from build123d import *

# Parameters (mm, degrees)
SKETCH1_R          = 20
EXTRUDE1_DEPTH     = 40
SKETCH2_R          = 2.5
SKETCH4_R          = 18
CUT_EXTRUDE1_DEPTH = 38
FILLET1_R          = 0.75
FILLET2_R          = 0.75
SCALE1_SCALE       = 2.5
SCALE2_SCALE       = 1.2


with BuildPart() as part:
    # Sketch1 → Extrude1 (new body)
    with BuildSketch(Plane(origin=(0, 0, 0), x_dir=(1, 0, 0), z_dir=(0, 1, 0))):
        Circle(SKETCH1_R)
    extrude(amount=EXTRUDE1_DEPTH)

    # Sweep1: sweep along a path in Sketch3
    with BuildLine(Plane.XY) as sweep1_path:
        Line((0, 30.773001508), (21.65, 30.773001508))
        ThreePointArc((21.65, 30.773001508), (33.01, 19.413001508), (21.65, 8.053001508))
        Line((21.65, 8.053001508), (0, 8.053001508))
    # Sketch2 → Sweep1 (sweep)
    with BuildSketch(Plane(origin=(0, 0, 0), x_dir=(0, 0, -1), z_dir=(1, 0, 0))):
        with Locations((0, 33.273001508)):
            Circle(SKETCH2_R)
    sweep(path=sweep1_path.line)

    # Sketch4 → Cut-Extrude1 (cut)
    with BuildSketch(Plane(origin=(0, 40, 0), x_dir=(-1, 0, 0), z_dir=(0, 1, 0))):
        Circle(SKETCH4_R)
    extrude(amount=-CUT_EXTRUDE1_DEPTH, mode=Mode.SUBTRACT)

    # Fillet1
    fillet1_edges = [part.edges().sort_by_distance(p)[0] for p in [
        (18, 40, 0),
        (-20, 40, 0),
    ]]
    fillet(fillet1_edges, radius=FILLET1_R)

    # Fillet2
    fillet2_edges = [part.edges().sort_by_distance(p)[0] for p in [
        (18, 2, 0),
    ]]
    fillet(fillet2_edges, radius=FILLET2_R)


with BuildPart() as part_1:
    # Scale1: scaled about (2.200885097, 16.795438051, 2.029e-06)
    add(part.part.scale(SCALE1_SCALE).moved(Location((-3.301327645, -25.193157077, -3.043e-06))))


with BuildPart() as part_2:
    # Scale2: scaled about (2.200885096, 16.795438052, 2.029e-06)
    add(part_1.part.scale(SCALE2_SCALE).moved(Location((-0.440177019, -3.35908761, -4.06e-07))))


solid = part_2.part
CAD build for the part. Positions are in the model's coordinates, mm. A direction names the side the tool comes from. Give positions to 0.01 mm unless a question says otherwise; leave off trailing zeros. Put each result on its own line as item: value.
(1) Tool access for faces 4 (the cylindrical face through (57.876, 73.664, 0.976)), 5 (the flat face through (-4, -27.591, 1)): list every direction of +Z, -Z, +X, -X, +Y, -Y with a clear straight run to the whole face (end or side of a thin tool).
Working result:
face 4: none
face 5: +Y
(2) Drop flat-ended pins along their axis: pin 1 Ø10 at (x, y) = (23, -21) entering from -Z; pin 2 Ø12 at (y, z) = (26.5, -14.5) entering from +X; pin 3 Ø8 at (x, y) = (5, 51.5) entering from +Z. Give the stop position or say it passes through.
Working result:
pin 1: z = -55.66
pin 2: x = 54.99
pin 3: z = 59.76
(3) Saw through at A-A (y = -5). Count the separate pieces of the cut face and the enclosed holes in it, then the cut area to 3 significant figures.
Working result:
separate pieces: 2
enclosed holes: 1
area: 2,410 mm^2
(4) Wall check: L1, parallel to X at y = -25.5, z = 1; L2, parallel to X at y = 41.5, z = 37; L3, parallel to Z at x = 9, y = 18.5. Give the ranges that are in metal, low to high.
Working result:
L1: -64.39 to -58.39, 49.58 to 55.59
L2: -51.64 to -43.73, 34.93 to 42.83
L3: -58.48 to -52.31, 52.31 to 58.48
(5) Pull direction Y, two halves, no side cores. Call faces 1 (the cylindrical face through (57.8, -17.262, 7.493)), 2 (the flat face through (8.2, 86.409, 55.3)), 3 (the flat face through (-5, -33.591, -1)): released by +Y, released by -Y, zero draft, split by the parting line, or undercut.
Working result:
face 1: undercut
face 2: released by +Y
face 3: released by -Y
